```python
from build123d import *

# Parameters (mm, degrees)
BOSS_EXTRUDE1_DEPTH = 5.715


with BuildPart() as part:
    # Model → Boss-Extrude1 (new body)
    with BuildSketch(Plane.XY):
        Polygon((863.263977742, 22.860238699), (866.236815782, 22.860238699), (866.236815782, 28.575245224), (877.667537494, 28.575245224), (877.667537494, 22.860238699), (889.098259207, 22.860238699), (889.098259207, 28.575245224), (900.528980919, 28.575245224), (900.528980919, 22.860238699), (911.95615932, 22.860238699), (911.95615932, 28.575245224), (923.386881032, 28.575245224), (923.386881032, 22.860238699), (934.817602745, 22.860238699), (934.817602745, 28.575245224), (946.248324457, 28.575245224), (946.248324457, 22.860238699), (957.679046169, 22.860238699), (957.679046169, 28.575245224), (969.10622457, 28.575245224), (969.10622457, 22.860238699), (972.082605921, 22.860238699), (972.082605921, 28.575245224), (972.082605921, 288.575408216), (972.082605921, 294.290414741), (969.10622457, 294.290414741), (969.10622457, 288.575408216), (957.679046169, 288.575408216), (957.679046169, 294.290414741), (946.248324457, 294.290414741), (946.248324457, 288.575408216), (934.817602745, 288.575408216), (934.817602745, 294.290414741), (923.386881032, 294.290414741), (923.386881032, 288.575408216), (911.95615932, 288.575408216), (911.95615932, 294.290414741), (900.528980919, 294.290414741), (900.528980919, 288.575408216), (889.098259207, 288.575408216), (889.098259207, 294.290414741), (877.667537494, 294.290414741), (877.667537494, 288.575408216), (866.236815782, 288.575408216), (866.236815782, 294.290414741), (863.263977742, 294.290414741), (863.263977742, 288.575408216), (863.263977742, 265.715382116), (863.653299053, 262.757291337), (864.794688151, 260.000375591), (866.610192193, 257.633089424), (868.975795287, 255.816433806), (871.344498779, 254.00013252), (873.160445734, 251.633200684), (874.303606488, 248.876284937), (874.694699455, 245.918194159), (874.694699455, 71.232246682), (874.302277747, 68.274290549), (873.160445734, 65.517240157), (871.344498779, 63.150485487), (868.975795287, 61.334361366), (866.610192193, 59.517571103), (864.794688151, 57.150419581), (863.653299053, 54.393369189), (863.263977742, 51.435413056), (863.263977742, 28.575245224), align=None)
        Polygon((880.410060311, 272.875350921), (880.410060311, 278.590357446), (886.121877856, 278.590357446), (886.121877856, 267.160344396), (880.410060311, 267.160344396), align=None, mode=Mode.SUBTRACT)
        Polygon((880.410060311, 250.015324821), (880.410060311, 255.730331346), (886.121877856, 255.730331346), (886.121877856, 244.300318296), (880.410060311, 244.300318296), align=None, mode=Mode.SUBTRACT)
        Polygon((880.410060311, 227.155298721), (880.410060311, 232.870305246), (886.121877856, 232.870305246), (886.121877856, 221.440292196), (880.410060311, 221.440292196), align=None, mode=Mode.SUBTRACT)
        Polygon((880.410060311, 204.295272621), (880.410060311, 210.010279146), (886.121877856, 210.010279146), (886.121877856, 198.580266096), (880.410060311, 198.580266096), align=None, mode=Mode.SUBTRACT)
        Polygon((880.410060311, 181.435246521), (880.410060311, 187.150253046), (886.121877856, 187.150253046), (886.121877856, 175.720239996), (880.410060311, 175.720239996), align=None, mode=Mode.SUBTRACT)
        Polygon((880.410060311, 158.575220421), (880.410060311, 164.290226946), (886.121877856, 164.290226946), (886.121877856, 152.860213896), (880.410060311, 152.860213896), align=None, mode=Mode.SUBTRACT)
        Polygon((880.410060311, 135.71519432), (880.410060311, 141.430200846), (886.121877856, 141.430200846), (886.121877856, 130.000187795), (880.410060311, 130.000187795), align=None, mode=Mode.SUBTRACT)
        Polygon((880.410060311, 112.85516822), (880.410060311, 118.570174745), (886.121877856, 118.570174745), (886.121877856, 107.140161695), (880.410060311, 107.140161695), align=None, mode=Mode.SUBTRACT)
        Polygon((880.410060311, 89.99514212), (880.410060311, 95.710148645), (886.121877856, 95.710148645), (886.121877856, 84.280135595), (880.410060311, 84.280135595), align=None, mode=Mode.SUBTRACT)
        Polygon((880.410060311, 67.13511602), (880.410060311, 72.850122545), (886.121877856, 72.850122545), (886.121877856, 61.420109495), (880.410060311, 61.420109495), align=None, mode=Mode.SUBTRACT)
        Polygon((880.410060311, 44.27508992), (880.410060311, 49.990096445), (886.121877856, 49.990096445), (886.121877856, 38.560083395), (880.410060311, 38.560083395), align=None, mode=Mode.SUBTRACT)
    extrude(amount=BOSS_EXTRUDE1_DEPTH)


solid = part.part
```
Verification items for the finished model (mm, model axes). A direction names the side the tool comes from. Give positions to 0.01 mm unless a question says otherwise; leave off trailing zeros. Order: outer loops, then holes, each group sorted by start corner. A loop starts at its lowest first (then second) coordinate and runs counter-clockwise, first axis right, second up. Notation, with made-up numbers: M 8.5,-16.75 L 48.5,-16.75 A16 cw 48.5,-9.75 Z; hole C 31.25,42 d3. An arc over 180 degrees is marked long. Return JSON: item names as keys, results as strings. Group by question number.
1) Section check D-D on x = 920. Record the cut outline in (y, z) (3 decimals), and give its area (3 significant figures).
2) Access from +Z, -Z, +X, -X, +Y, -Y to the whole of each face (thin tool, end or side, straight path). Record for faces 4 (the face through (880.41, 113, 3)), 5 (the face through (969.106, 291, 3)), 6 (the face through (934.818, 26, 3)).
3) Mould release check, pull along X, two halves, no side actions. Record for faces 1 (the face through (934.818, 291, 3)), 2 (the face through (883, 22.86, 3)), 3 (the face through (874.695, 160, 3)): pulls with the +X half, pulls with the -X half, needs draft (parallel to the pull), parting line crosses it, or undercut.
4) Go/stop test with flat-tipped pins: pin 1 Ø3 at (y, z) = (91.5, 4) entering from -X; pin 2 Ø3 at (x, z) = (893, 2) entering from +Y; pin 3 Ø3 at (x, z) = (894, 3) entering from -Y. Record where each tip stops, or that it passes through.
5) Scan lines: line 1 (X direction, y = 45.5, z = 1.3); line 2 (X direction, y = 227.5, z = 2.2); line 3 (Y direction, x = 940, z = 3). Record each from-to range of solid material in increasing order.
6) Section check A-A on y = 202.5. Record the cut outline in (x, z) (3 decimals).
7) Section check B-B on x = 883. Give the number of separate pieces and of enclosed holes in the cut face, and give its area (3 significant figures).
Answer block:
{
 "1": {"outline": "M 28.575,0 L 288.575,0 L 288.575,5.715 L 28.575,5.715 Z", "area": "1,490 mm^2"},
 "2": {"face 4": "+Z, -Z", "face 5": "+Z, -Z, +Y", "face 6": "+Z, -Z, -Y"},
 "3": {"face 1": "undercut", "face 2": "needs draft", "face 3": "pulls with the -X half"},
 "4": {"pin 1": "stops at x = 874.69", "pin 2": "stops at y = 288.58", "pin 3": "stops at y = 28.58"},
 "5": {"line 1": "x = 863.26 to 880.41, 886.12 to 972.08", "line 2": "x = 874.69 to 880.41, 886.12 to 972.08", "line 3": "y = 28.58 to 288.58"},
 "6": {"outline": "M 874.695,0 L 880.41,0 L 880.41,5.715 L 874.695,5.715 Z; M 886.122,0 L 972.083,0 L 972.083,5.715 L 886.122,5.715 Z"},
 "7": {"separate pieces": "12", "enclosed holes": "0", "area": "833 mm^2"}
}
